```python
from build123d import *

# Parameters (mm, degrees)
SKETCH1_W           = 20
SKETCH1_H           = 20
BOSS_EXTRUDE1_DEPTH = 400
SKETCH2_R           = 3
CUT_EXTRUDE1_DEPTH  = 401.249921924
CUT_EXTRUDE2_DEPTH  = 401.249921924
CIRPATTERN1_COUNT   = 4


with BuildPart() as part:
    # Sketch1 → Boss-Extrude1 (new body)
    with BuildSketch(Plane(origin=(0, 0, 0), x_dir=(0, 0, -1), z_dir=(1, 0, 0))):
        Rectangle(SKETCH1_W, SKETCH1_H)
    extrude(amount=BOSS_EXTRUDE1_DEPTH)

    # Sketch2 → Cut-Extrude1 (cut, through all)
    with BuildSketch(Plane(origin=(400, 0, 0), x_dir=(0, 0, -1), z_dir=(1, 0, 0))):
        Circle(SKETCH2_R)
    extrude(amount=-CUT_EXTRUDE1_DEPTH, mode=Mode.SUBTRACT)

    # Sketch2_3 → Cut-Extrude2 (cut, through all)
    with BuildSketch(Plane(origin=(400, 0, 0), x_dir=(0, 0, -1), z_dir=(1, 0, 0))):
        Polygon((0, 10), (0, 5), (3.5, 5), (6, 7), (6, 8.5), (4.5, 8.5), (4.5, 10), align=None)
        Polygon((-3.5, 5), (0, 5), (0, 10), (-4.5, 10), (-4.5, 8.5), (-6, 8.5), (-6, 7), align=None)
    cut_extrude2 = extrude(amount=-CUT_EXTRUDE2_DEPTH, mode=Mode.SUBTRACT)

    # CirPattern1: Cut-Extrude2 ×4 about axis
    cirpattern1_axis = Axis((0, 0, 0), (1, 0, 0))
    for i in range(1, CIRPATTERN1_COUNT):
        add(cut_extrude2.rotate(cirpattern1_axis, i * 360 / CIRPATTERN1_COUNT), mode=Mode.SUBTRACT)


solid = part.part
```
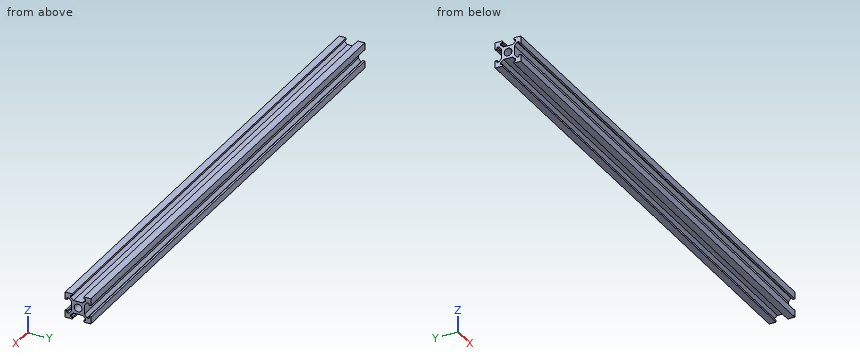
Geometry: final body of the model. Coordinates: model frame, mm. Give positions to 0.01 mm unless a question says otherwise; leave off trailing zeros. Order: outer loops, then holes, each group sorted by start corner. A loop starts at its lowest first (then second) coordinate and runs counter-clockwise, first axis right, second up. Notation, with made-up numbers: (52.5, -37.5) -> (73.5, -37.5) arc R24 cw to (73.5, -18.5) -> close; hole circle Ø5 at (41, 79.5). An arc over 180 degrees is marked (long way). Write each question's results on one line, items separated by ' | '. Start each with the question number.
1) Section A-A (z = 0). Return loops of the section in (x, y).
2) Line query: line 1 (Z direction, x = 130, y = 8); line 2 (Y direction, x = 83.5, z = 0); line 3 (Z direction, x = 220.5, y = 2). Output: solid intervals per line, ascending. Write a range as from..to.
3) First-contact query: pin 1 (7.5 mm diameter, centred on x = 181, y = 0, fed in from +Z); pin 2 (3 mm diameter, centred on x = 239, y = 0.5, fed in from +Z); pin 3 (5.5 mm diameter, centred on x = 244, y = 1.5, fed in from -Z). Flat tips, straight axial feed; report the tip coordinate or a pass-through.
Calculated:
1) outline: (0, -5) -> (400, -5) -> (400, -3) -> (0, -3) -> close; (0, 3) -> (400, 3) -> (400, 5) -> (0, 5) -> close
2) line 1: -10..-6, 6..10 | line 2: -5..-3, 3..5 | line 3: -5..-2.24, 2.24..5
3) pin 1: z = 5.2 | pin 2: z = 5 | pin 3: z = -5.6
